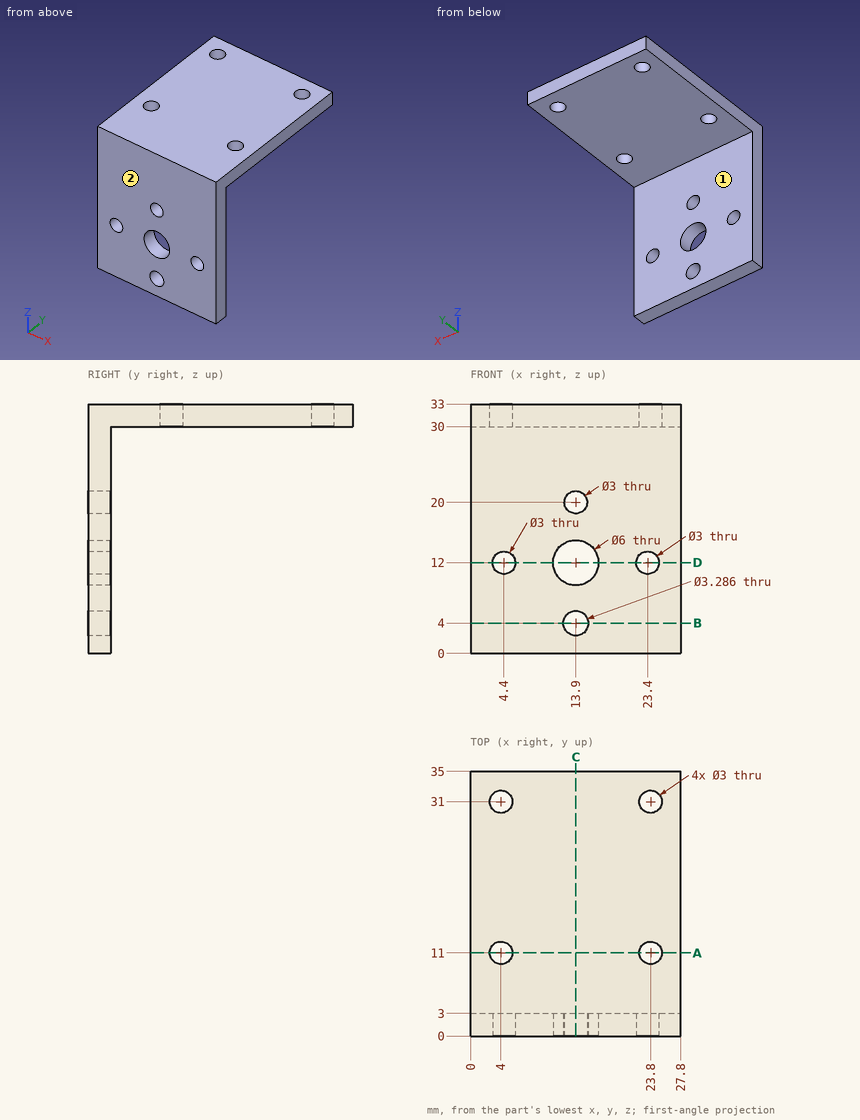
The figure shows three views and two pictorial views of one solid part (mm, origin at its lowest corner). Answer the questions. A direction names the side the tool comes from. Round coordinates to 2 decimals unless told otherwise and drop trailing zeros. Loops run counter-clockwise (first coordinate to the right, second up) from the corner with the lowest first, then second, coordinate; pieces in that order, holes last. Notation, with made-up numbers: (-8.5, 36.25) - (12.5, 36.25) arc R20 ccw to (12.5, 51.25) - close; hole circle Ø11 at (9, 60). An arc over 180 degrees is marked (long way). Use one line per item in the form item = value. Start each with the question number.
(1) Find section A-A on y = 11. Determine the outline of the cut face in (x, z), and give its area (3 significant figures).
(2) Flat-ended cylindrical pins translate along their axes: P1, Ø1.8, axis at x = 23.4, z = 12, coming from the +Y side; P2, Ø5, axis at x = 23.8, y = 11, coming from the -Z side; P3, Ø5, axis at x = 6, z = 7.5, coming from the +Y side. Find the tip coordinate at first contact, or state that the pin passes through.
(3) Consider line 1 (Y direction, x = 23.8, z = 31.15); line 2 (X direction, y = 1.4, z = 4); line 3 (Y direction, x = 1.5, z = 22). Determine where each line is inside the solid, lowest interval first.
(4) Find section C-C on x = 13.9. Determine the outline of the cut face in (y, z).
(5) Find section D-D on z = 12. Determine the outline of the cut face in (x, y).
(6) Find section B-B on z = 4. Determine the outline of the cut face in (x, y).
(7) Which of the six approach directions +Z, -Z, +X, -X, +Y, -Y give full straight-line access (tool end or side, diameter ignored) to the marked faces 1 and 2?
Answer list:
q1.outline = (0, 30) - (2.5, 30) - (2.5, 33) - (0, 33) - close; (5.5, 30) - (22.3, 30) - (22.3, 33) - (5.5, 33) - close; (25.3, 30) - (27.8, 30) - (27.8, 33) - (25.3, 33) - close
q1.area = 65.4 mm^2
q2.P1 = through
q2.P2 = 30
q2.P3 = 3
q3.line_1 = 0 to 9.5, 12.5 to 29.5, 32.5 to 35
q3.line_2 = 0 to 12.26, 15.54 to 27.8
q3.line_3 = 0 to 3
q4.outline = (0, 0) - (3, 0) - (3, 2.36) - (0, 2.36) - close; (0, 5.64) - (3, 5.64) - (3, 9) - (0, 9) - close; (0, 15) - (3, 15) - (3, 18.5) - (0, 18.5) - close; (0, 21.5) - (3, 21.5) - (3, 30) - (35, 30) - (35, 33) - (0, 33) - close
q5.outline = (0, 0) - (2.9, 0) - (2.9, 3) - (0, 3) - close; (5.9, 0) - (10.9, 0) - (10.9, 3) - (5.9, 3) - close; (16.9, 0) - (21.9, 0) - (21.9, 3) - (16.9, 3) - close; (24.9, 0) - (27.8, 0) - (27.8, 3) - (24.9, 3) - close
q6.outline = (0, 0) - (12.26, 0) - (12.26, 3) - (0, 3) - close; (15.54, 0) - (27.8, 0) - (27.8, 3) - (15.54, 3) - close
q7.face_1 = -Z, +X, -X, +Y
q7.face_2 = +Z, -Z, +X, -X, -Y
